Part model, mm, in its own coordinate system. Face numbers are marked on the shaded views. A direction names the side the tool comes from. Coordinates: 2 decimals unless noted, no trailing zeros. Loops run counter-clockwise (first coordinate to the right, second up) from the corner with the lowest first, then second, coordinate; pieces in that order, holes last. Notation, with made-up numbers: M 33,-7.5 L 80,-7.5 A25 ccw 80,22.5 Z; hole C -16.5,-3 d8. An arc over 180 degrees is marked long. Use a Markdown table: item, result. Add a question column.
1) Band-saw the part on C-C (y = 19). List the corners of the cut face in (x, z).
2) Band-saw the part on B-B (x = 0). List the corners of the cut face in (y, z).
3) Wall check: probe 1 along Z at (x, y) = (0, 12.25); probe 2 along Z at (x, y) = (8.15, 19); probe 3 along Y at (x, z) = (7.1, 0). Give the ranges that are in metal, low to high. Write a range as from..to.
4) Tool access for the marked faces 1, 2 and 3: list every direction of +Z, -Z, +X, -X, +Y, -Y with a clear straight run to the whole face (end or side of a thin tool).
5) Band-saw the part on A-A (y = 8). List the corners of the cut face in (x, z), plus the area to 3 significant figures.
6) Pin check, flat tips, straight feed: pin 1 Ø1 at (x, z) = (-3, -0.5) entering from -Y; pin 2 Ø11 at (y, z) = (19, 0) entering from +X. Stop position of each tip, or through.
7) Band-saw the part on D-D (x = 11). List the corners of the cut face in (y, z).
8) Pull direction Y, two halves, no side cores. Call the marked faces 4, 5 and 6: released by +Y, released by -Y, zero draft, split by the parting line, or undercut.
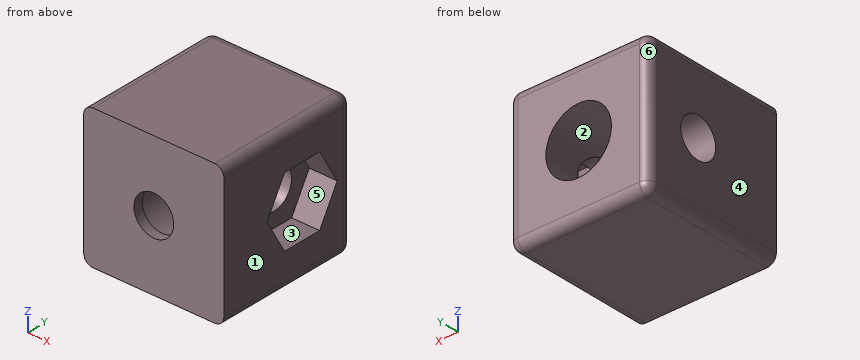
Autodesk Inventor part; units mm, degrees
ref_plane "YZ Plane" through (0, 0, 0) normal (1, 0, 0) x (0, 1, 0)
ref_plane "XZ Plane" through (0, 0, 0) normal (0, 1, 0) x (-1, 0, 0)
ref_plane "XY Plane" through (0, 0, 0) normal (0, 0, 1) x (1, 0, 0)
sketch "Sketch1" plane through (0, 0, 0) normal (0, 1, 0) x (-1, 0, 0)
  line L0 (-15, 15) -> (15, 15)
  line L1 (15, 15) -> (15, -15)
  line L2 (15, -15) -> (-15, -15)
  line L3 (-15, -15) -> (-15, 15)
  line L4 (-15, 15) -> (15, -15) construction
  line L5 (15, 15) -> (-15, -15) construction
  point P0 (0, 0)
  dimension "d0" = 30
  dimension "d1" = 30
extrude "Extrusion1" add sketch "Sketch1" along normal blind 11
sketch "Sketch2" plane through (0, 11, 0) normal (0, 1, 0) x (1, 0, 0)
  circle A0 centre (0, 0) radius 7
  dimension "d4" = 14
extrude "Extrusion2" cut sketch "Sketch2" against normal blind 9
sketch "Sketch3" plane through (0, 11, 0) normal (0, 1, 0) x (1, 0, 0)
  circle A0 centre (0, 0) radius 7
  line L0 (-15, -15) -> (15, -15)
  line L1 (15, -15) -> (15, 15)
  line L2 (15, 15) -> (-15, 15)
  line L3 (-15, 15) -> (-15, -15)
extrude "Extrusion3" add sketch "Sketch3" along normal blind 20
sketch "Sketch4" plane through (15, 0, 15) normal (1, 0, 0) x (0, 0, -1)
  circle A0 centre (15, 19) radius 4
  line L0 (0, 31) -> (30, 31)
  line L1 (15, 27.5448) -> (22.4, 23.2724)
  line L2 (22.4, 23.2724) -> (22.4, 14.7276)
  line L3 (22.4, 14.7276) -> (15, 10.4552)
  line L4 (15, 10.4552) -> (7.6, 14.7276)
  line L5 (7.6, 14.7276) -> (7.6, 23.2724)
  line L6 (7.6, 23.2724) -> (15, 27.5448)
  circle A1 centre (15, 19) radius 7.4
  point P0 (15, 0)
  dimension "d9" = 8
  dimension "d10" = 12
  dimension "d22" = 14.8
extrude "Extrusion4" cut sketch "Sketch4" against normal blind 6 contours A0 | L1 A1 L6 | L1 L2 A1 | A1 | A1 L5 L6 | L2 L3 A1 | A1 L4 L5 | L3 L4 A1
sketch "Sketch5" plane through (9, 0, 15) normal (1, 0, 0) x (0, 0, -1)
  circle A0 centre (15, 19) radius 4.25
  line L0 (0, 31) -> (30, 31)
  point P0 (15, 0)
  dimension "d14" = 8.5
  dimension "d20" = 12
extrude "Extrusion5" cut sketch "Sketch5" against normal through all
sketch "Sketch6" plane through (0, 2, 0) normal (0, 1, 0) x (1, 0, 0)
  circle A0 centre (0, 0) radius 4.25
  dimension "d17" = 8.5
extrude "Extrusion6" cut sketch "Sketch6" against normal through all
fillet "Fillet1" radius 2 4 edges at (15, 15.5, -15) (-15, 15.5, -15) (-15, 15.5, 15) (15, 15.5, 15)
fillet "Fillet2" radius 2 8 edges at (14.4142, 31, 14.4142) (15, 31, 0) (14.4142, 31, -14.4142) (0, 31, -15) (-14.4142, 31, -14.4142) (-15, 31, 0) (-14.4142, 31, 14.4142) (0, 31, 15)
properties part number "Spoolsupport"
Entries:
| question | item | result |
|---|---|---|
| 1 | outline | M -15,-13 A2 ccw -13,-15 L 13,-15 A2 ccw 15,-13 L 15,-7.4 L 9,-7.4 L 9,-4.25 L 5.56,-4.25 A7 cw -5.56,-4.25 L -15,-4.25 Z; M -15,4.25 L -5.56,4.25 A7 cw 5.56,4.25 L 9,4.25 L 9,7.4 L 15,7.4 L 15,13 A2 ccw 13,15 L -13,15 A2 ccw -15,13 Z |
| 2 | outline | M 0,-15 L 29,-15 A2 ccw 31,-13 L 31,-7 L 2,-7 L 2,-4.25 L 0,-4.25 Z; M 0,4.25 L 2,4.25 L 2,7 L 31,7 L 31,13 A2 ccw 29,15 L 0,15 Z |
| 3 | probe 1 | -15..-7, 7..15 |
| 3 | probe 2 | -15..-4.25, 4.25..15 |
| 3 | probe 3 | 0..14.75, 23.25..31 |
| 4 | face 1 | +Z, -Z, +X, +Y, -Y |
| 4 | face 2 | +Y |
| 4 | face 3 | +X |
| 5 | outline | M -15,-13 A2 ccw -13,-15 L 13,-15 A2 ccw 15,-13 L 15,13 A2 ccw 13,15 L -13,15 A2 ccw -15,13 Z; hole C 0,0 d14 |
| 5 | area | 743 mm2 |
| 6 | pin 1 | through |
| 6 | pin 2 | x = 9 |
| 7 | outline | M 0,-15 L 29,-15 A2 ccw 31,-13 L 31,13 A2 ccw 29,15 L 0,15 Z; hole M 10.46,0 L 14.73,-7.4 L 23.27,-7.4 L 27.54,0 L 23.27,7.4 L 14.73,7.4 Z |
| 8 | face 4 | zero draft |
| 8 | face 5 | undercut |
| 8 | face 6 | released by +Y |
